from build123d import *

# Parameters (mm, degrees)
PAD001_DEPTH    = 3.3
SKETCH_W        = 80
SKETCH_H        = 80
PAD_DEPTH       = 10
SKETCH001_R     = 11.05
POCKET_DEPTH    = 7
SKETCH002_R     = 5
POCKET001_DEPTH = 3.001
SKETCH003_R     = 13.05
POCKET002_DEPTH = 0.9
POCKET003_DEPTH = 7
POCKET004_DEPTH = 3.001
POCKET005_DEPTH = 10.001
SKETCH009_W     = 8
SKETCH009_H     = 12
SKETCH009_W_2   = 12
SKETCH009_H_2   = 8
POCKET008_DEPTH = 10.001
SKETCH010_R     = 2.1
POCKET009_DEPTH = 9
SKETCH011_R     = 2.1
POCKET010_DEPTH = 9
SKETCH012_R     = 2.1
POCKET011_DEPTH = 8.5
POCKET012_DEPTH = 2.55
POCKET013_DEPTH = 2.55
SKETCH017_R     = 5.4
SKETCH017_R_2   = 5
PAD002_DEPTH    = 7
SKETCH018_R     = 11.45
SKETCH018_R_2   = 11.05
PAD003_DEPTH    = 0.9
SKETCH019_R     = 9
SKETCH019_R_2   = 8.6
PAD004_DEPTH    = 7


with BuildPart() as pad001:
    # Sketch016 → Pad001 (new body)
    with BuildSketch(Plane.XZ.offset(-29)):
        Polygon((-25.475, 7.03516), (-29, 9.070319), (-32.525, 7.03516), (-32.525, 2.96484), (-32.525, 0), (-25.475, 0), align=None)
        Polygon((32.525, 7.03516), (29, 9.070319), (25.475, 7.03516), (25.475, 2.96484), (25.475, 0), (32.525, 0), align=None)
    extrude(amount=PAD001_DEPTH)


with BuildPart() as obj1:
    # Sketch → Pad (new body)
    with BuildSketch(Plane.XY):
        Rectangle(SKETCH_W, SKETCH_H)
    extrude(amount=PAD_DEPTH)

    # Sketch001 → Pocket (cut)
    with BuildSketch(Plane.XY.offset(10)):
        with Locations((0, 25.95)):
            Circle(SKETCH001_R)
    extrude(amount=-POCKET_DEPTH, mode=Mode.SUBTRACT)

    # Sketch002 → Pocket001 (cut, through all)
    with BuildSketch(Plane.XY.offset(3)):
        with Locations((0, 25.95)):
            Circle(SKETCH002_R)
    extrude(amount=-POCKET001_DEPTH, mode=Mode.SUBTRACT)

    # Sketch003 → Pocket002 (cut)
    with BuildSketch(Plane.XY.offset(10)):
        with Locations((0, 25.95)):
            Circle(SKETCH003_R)
    extrude(amount=-POCKET002_DEPTH, mode=Mode.SUBTRACT)

    # Sketch004 → Pocket003 (cut)
    with BuildSketch(Plane(origin=(0, 0, 0), x_dir=(1, 0, 0), z_dir=(0, 0, -1))):
        with BuildLine():
            ThreePointArc((-20, 10), (0, -10), (20, 10))
            Line((20, 40), (20, 10))
            Line((20, 40), (-20, 40))
            Line((-20, 40), (-20, 10))
        make_face()
    extrude(amount=-POCKET003_DEPTH, mode=Mode.SUBTRACT)

    # Sketch005 → Pocket004 (cut, through all)
    with BuildSketch(Plane(origin=(0, 0, 7), x_dir=(1, 0, 0), z_dir=(0, 0, -1))):
        with BuildLine():
            ThreePointArc((3, 16), (0, 19), (-3, 16))
            Line((-3, 16), (-3, 8))
            ThreePointArc((-3, 8), (0, 5), (3, 8))
            Line((3, 16), (3, 8))
        make_face()
        with BuildLine():
            ThreePointArc((13.85, 16), (12.25, 17.6), (10.65, 16))
            Line((10.65, 16), (10.65, 8))
            ThreePointArc((10.65, 8), (12.25, 6.4), (13.85, 8))
            Line((13.85, 16), (13.85, 8))
        make_face()
        with BuildLine():
            ThreePointArc((-10.65, 16), (-12.25, 17.6), (-13.85, 16))
            Line((-13.85, 16), (-13.85, 8))
            ThreePointArc((-13.85, 8), (-12.25, 6.4), (-10.65, 8))
            Line((-10.65, 16), (-10.65, 8))
        make_face()
    extrude(amount=-POCKET004_DEPTH, mode=Mode.SUBTRACT)

    # Sketch006 → Pocket005 (cut, through all)
    with BuildSketch(Plane.XY.offset(10)):
        Polygon((-40, 40), (-35, 40), (-35, -35), (35, -35), (35, 40), (40, 40), (40, -40), (35, -40), (-35, -40), (-40, -40), align=None)
    extrude(amount=-POCKET005_DEPTH, mode=Mode.SUBTRACT)

    # Sketch009 → Pocket008 (cut, through all)
    with BuildSketch(Plane.XY.offset(10)):
        with Locations((-31, 9)):
            Rectangle(SKETCH009_W, SKETCH009_H)
        with Locations((31, 9)):
            Rectangle(SKETCH009_W, SKETCH009_H)
        with Locations((-31, -21)):
            Rectangle(SKETCH009_W, SKETCH009_H)
        with Locations((31, -21)):
            Rectangle(SKETCH009_W, SKETCH009_H)
        with Locations((-29, 36)):
            Rectangle(SKETCH009_W_2, SKETCH009_H_2)
        with Locations((29, 36)):
            Rectangle(SKETCH009_W_2, SKETCH009_H_2)
    extrude(amount=-POCKET008_DEPTH, mode=Mode.SUBTRACT)

    # Sketch010 → Pocket009 (cut)
    with BuildSketch(Plane(origin=(-27, 0, 0), x_dir=(0, -1, 0), z_dir=(-1, 0, 0))):
        with Locations((-9, 5)):
            Circle(SKETCH010_R)
        with Locations((21, 5)):
            Circle(SKETCH010_R)
    extrude(amount=-POCKET009_DEPTH, mode=Mode.SUBTRACT)

    # Sketch011 → Pocket010 (cut)
    with BuildSketch(Plane.YZ.offset(27)):
        with Locations((-21, 5)):
            Circle(SKETCH011_R)
        with Locations((9, 5)):
            Circle(SKETCH011_R)
    extrude(amount=-POCKET010_DEPTH, mode=Mode.SUBTRACT)

    # Sketch012 → Pocket011 (cut)
    with BuildSketch(Plane(origin=(0, 32, 0), x_dir=(-1, 0, 0), z_dir=(0, 1, 0))):
        with Locations((-29, 5)):
            Circle(SKETCH012_R)
        with Locations((29, 5)):
            Circle(SKETCH012_R)
    extrude(amount=-POCKET011_DEPTH, mode=Mode.SUBTRACT)

    # Sketch013 → Pocket012 (cut, symmetric)
    with BuildSketch(Plane(origin=(20, 0, 0), x_dir=(0, -1, 0), z_dir=(-1, 0, 0))):
        Polygon((-5.475, 7.03516), (-9, 9.070319), (-12.525, 7.03516), (-12.525, 2.96484), (-12.525, 0), (-5.475, 0), align=None)
        Polygon((21, 9.070319), (17.475, 7.03516), (17.475, 2.96484), (17.475, 0), (24.525, 0), (24.525, 2.96484), (24.525, 7.03516), align=None)
    extrude(amount=POCKET012_DEPTH, both=True, mode=Mode.SUBTRACT)

    # Sketch014 → Pocket013 (cut, symmetric)
    with BuildSketch(Plane.YZ.offset(-20)):
        Polygon((-17.475, 7.03516), (-21, 9.070319), (-24.525, 7.03516), (-24.525, 2.96484), (-24.525, 0), (-17.475, 0), align=None)
        Polygon((12.525, 7.03516), (9, 9.070319), (5.475, 7.03516), (5.475, 2.96484), (5.475, 0), (12.525, 0), align=None)
    extrude(amount=POCKET013_DEPTH, both=True, mode=Mode.SUBTRACT)

    # Cut: cut Pad001
    add(pad001.part, mode=Mode.SUBTRACT)

    # Sketch017 → Pad002 (new body)
    with BuildSketch(Plane.XY.offset(3)):
        with Locations((0, 25.95)):
            Circle(SKETCH017_R)
        with Locations((0, 25.95)):
            Circle(SKETCH017_R_2, mode=Mode.SUBTRACT)
    extrude(amount=PAD002_DEPTH)

    # Sketch018 → Pad003 (new body)
    with BuildSketch(Plane.XY.offset(9.1)):
        with Locations((0, 25.95)):
            Circle(SKETCH018_R)
        with Locations((0, 25.95)):
            Circle(SKETCH018_R_2, mode=Mode.SUBTRACT)
    extrude(amount=PAD003_DEPTH)

    # Sketch019 → Pad004 (new body)
    with BuildSketch(Plane.XY.offset(3)):
        with Locations((0, 25.95)):
            Circle(SKETCH019_R)
        with Locations((-0.000162, 25.950293)):
            Circle(SKETCH019_R_2, mode=Mode.SUBTRACT)
    extrude(amount=PAD004_DEPTH)


solid = obj1.part
Here's how the part is built. I have some questions about the finished solid (model axes, mm). A direction names the side the tool comes from. Round coordinates to 2 decimals unless told otherwise and drop trailing zeros.
1. Suppose I cut it at A-A (x = 0). State how many separate pieces and enclosed holes the cut face has, and give its area (3 significant figures).
2. For faces 1 (the flat face through (31, -15, 5)), 2 (the flat face through (29, 25.7, 2.6)), 3 (the flat face through (-31, 3, 5)), 4 (the cylindrical face through (31.1, 30.52, 5.09)), which set-ups out of +Z, -Z, +X, -X, +Y, -Y let a thin tool reach every point of the face, with its end or its side?
3. I need wall thicknesses on L1, parallel to Y at x = 0, z = 6.75; L2, parallel to Y at x = -31, z = 2; L3, parallel to X at y = -29, z = 6. Which ranges of each line are inside material? Lowest first, please.
4. Will these pins go through, and if not, where does the flat tip stop? pin 1 Ø4 at (y, z) = (-21, 7.5) entering from +X; pin 2 Ø2.5 at (y, z) = (9, 5) entering from +X; pin 3 Ø4 at (x, y) = (26, 0) entering from -Z; pin 4 Ø3.5 at (x, z) = (29, 5.5) entering from +Y.
5. If we mould it in two halves opening along Y, with no side actions, what happens to faces 5 (the flat face through (-19.964, 7.262, 8.067)), 6 (the flat face through (0, 3, 10))? For each: released by +Y, released by -Y, zero draft, split by the parting line, or undercut.
Answer sheet:
1. separate pieces: 3
1. enclosed holes: 0
1. area: 217 mm2
2. face 1: +Z, -Z, +X
2. face 2: -Z
2. face 3: +Z, -Z, -X
2. face 4: +Y
3. L1: y = 10 to 14.9, 16.95 to 17.35, 20.55 to 20.95, 30.95 to 31.35, 34.55 to 34.95, 37 to 40
3. L2: y = -35 to -27, -15 to 3, 15 to 25.7, 29 to 32
3. L3: x = -35 to -20, 20 to 35
4. pin 1: stops at x = 27
4. pin 2: stops at x = 17.45
4. pin 3: stops at z = 0
4. pin 4: stops at y = 32
5. face 5: undercut
5. face 6: zero draft
